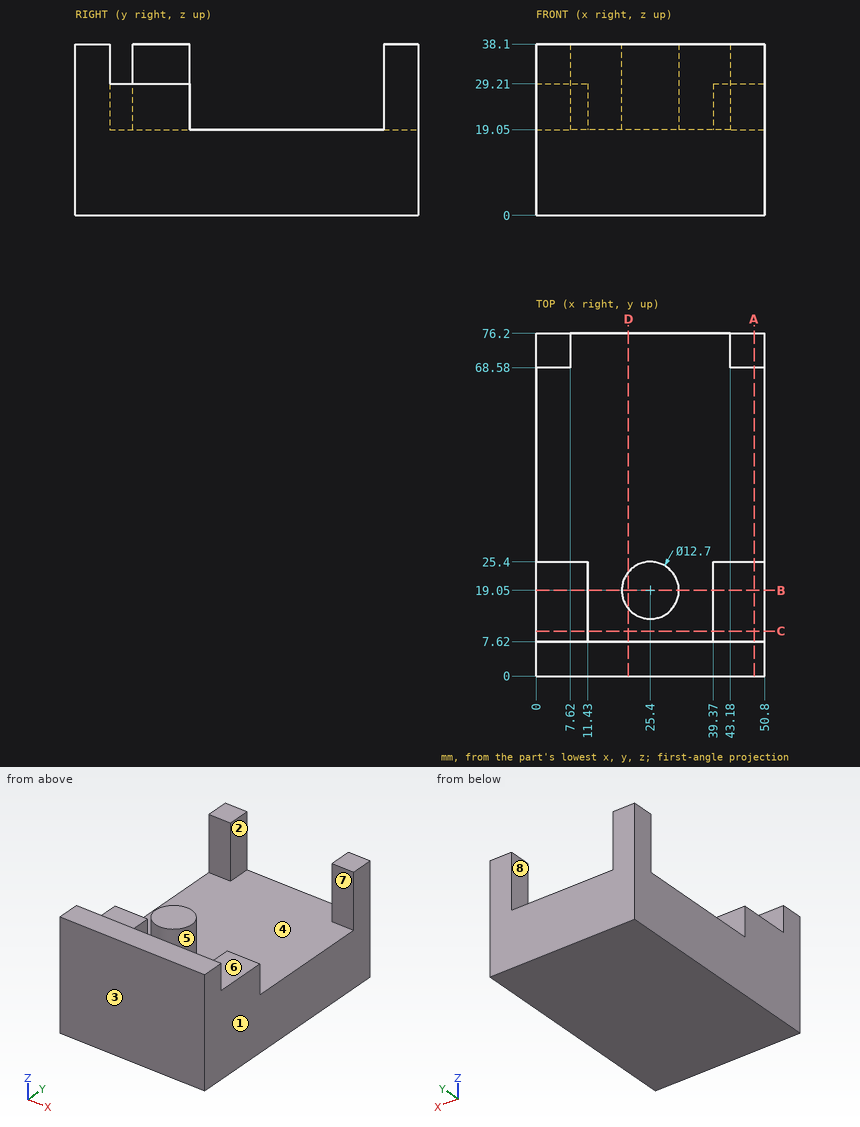
Here's the drawing with two shaded views (mm, measured from the low corner). I have some questions. A direction names the side the tool comes from. Coordinates: 2 decimals unless noted, no trailing zeros. Write each loop counter-clockwise with the first axis right and the second up, starting at its lowest first coordinate (ties: lowest second). Pieces come first, ordered by that corner, then holes. Notation, with made-up numbers: (29.25, 26) -> (84.25, 26) arc R11 ccw to (84.25, 32) -> close; hole circle Ø1 at (-8, -12.5). An arc over 180 degrees is marked (long way). Use a Markdown table: item, result. Add a question column.
(1) If we section it at B-B, the plane y = 19.05: Write out the boundary of the cut face in (x, z), and give its area (3 significant figures).
(2) For the marked faces 5, 6, 7 and 8, which set-ups out of +Z, -Z, +X, -X, +Y, -Y let a thin tool reach every point of the face, with its end or its side?
(3) If we section it at D-D, the plane x = 20.5: Write out the boundary of the cut face in (y, z).
(4) We'd pull the mould along X, two halves only. Please class the marked faces 1, 2, 3 and 4: +X half, -X half, draft (parallel to the pull), parting line (faces both ways), or undercut.
(5) If we section it at A-A, the plane x = 48.5: Write out the boundary of the cut face in (y, z), and give its area (3 significant figures).
(6) I'm going to push flat-ended pins straight in: P1, Ø3.5, axis at x = 6, y = 18.5, coming from the +Z side; P2, Ø15, axis at x = 15.5, z = 28.5, coming from the +Y side; P3, Ø4, axis at x = 14.5, z = 26, coming from the +Y side. Where does each tip first touch, or does it pass through?
(7) Please list where these lines run through material, in increasing order: line 1 (Z direction, x = 5, y = 11); line 2 (Z direction, x = 11.5, y = 56); line 3 (Y direction, x = 13.5, z = 32.5).
(8) If we section it at C-C, the plane y = 10: Write out the boundary of the cut face in (x, z).
Outcome:
| question | item | result |
|---|---|---|
| 1 | outline | (0, 0) -> (50.8, 0) -> (50.8, 29.21) -> (39.37, 29.21) -> (39.37, 19.05) -> (31.75, 19.05) -> (31.75, 38.1) -> (19.05, 38.1) -> (19.05, 19.05) -> (11.43, 19.05) -> (11.43, 29.21) -> (0, 29.21) -> close |
| 1 | area | 1,440 mm^2 |
| 2 | face 5 | +Z |
| 2 | face 6 | +Z, +X |
| 2 | face 7 | +Z, +X, -X |
| 2 | face 8 | +Z, +Y |
| 3 | outline | (0, 0) -> (76.2, 0) -> (76.2, 19.05) -> (23.09, 19.05) -> (23.09, 38.1) -> (15.01, 38.1) -> (15.01, 19.05) -> (7.62, 19.05) -> (7.62, 38.1) -> (0, 38.1) -> close |
| 4 | face 1 | +X half |
| 4 | face 2 | undercut |
| 4 | face 3 | draft |
| 4 | face 4 | undercut |
| 5 | outline | (0, 0) -> (76.2, 0) -> (76.2, 38.1) -> (68.58, 38.1) -> (68.58, 19.05) -> (25.4, 19.05) -> (25.4, 29.21) -> (7.62, 29.21) -> (7.62, 38.1) -> (0, 38.1) -> close |
| 5 | area | 1,920 mm^2 |
| 6 | P1 | stops at z = 29.21 |
| 6 | P2 | stops at y = 25.4 |
| 6 | P3 | stops at y = 7.62 |
| 7 | line 1 | z = 0 to 29.21 |
| 7 | line 2 | z = 0 to 19.05 |
| 7 | line 3 | y = 0 to 7.62 |
| 8 | outline | (0, 0) -> (50.8, 0) -> (50.8, 29.21) -> (39.37, 29.21) -> (39.37, 19.05) -> (11.43, 19.05) -> (11.43, 29.21) -> (0, 29.21) -> close |
